```python
from build123d import *

# Parameters (mm, degrees)
SKETCH1_R           = 23.5
BOSS_EXTRUDE1_DEPTH = 65
SKETCH2_R           = 7.5
BOSS_EXTRUDE2_DEPTH = 2
SKETCH3_R           = 2.5
BOSS_EXTRUDE3_DEPTH = 20
CUT_EXTRUDE2_START  = -7.5
CUT_EXTRUDE2_DEPTH  = 7.5


with BuildPart() as part:
    # Sketch1 → Boss-Extrude1 (new body)
    with BuildSketch(Plane(origin=(0, 0, 0), x_dir=(1, 0, 0), z_dir=(0, 1, 0))):
        with Locations(Location((0, 0, 0), (0, 0, 270))):
            Circle(SKETCH1_R)
    extrude(amount=BOSS_EXTRUDE1_DEPTH)

    # Sketch2 → Boss-Extrude2 (add)
    with BuildSketch(Plane(origin=(0, 65, 0), x_dir=(1, 0, 0), z_dir=(0, 1, 0))):
        with Locations(Location((0, 0, 0), (0, 0, 270))):
            Circle(SKETCH2_R)
    extrude(amount=BOSS_EXTRUDE2_DEPTH)

    # Sketch3 → Boss-Extrude3 (add)
    with BuildSketch(Plane(origin=(0, 67, 0), x_dir=(1, 0, 0), z_dir=(0, 1, 0))):
        with Locations(Location((0, 0, 0), (0, 0, 270))):
            Circle(SKETCH3_R)
    extrude(amount=BOSS_EXTRUDE3_DEPTH)

    # Sketch4 → Cut-Extrude2 (cut)
    with BuildSketch(Plane(origin=(0, 87, 0), x_dir=(1, 0, 0), z_dir=(0, 1, 0)).offset(CUT_EXTRUDE2_START)):
        with BuildLine():
            Line((0.591953549, 2.428907367), (0.591953549, -2.428907367))
            ThreePointArc((0.591953549, -2.428907367), (2.5, 0), (0.591953549, 2.428907367))
        make_face()
    extrude(amount=CUT_EXTRUDE2_DEPTH, mode=Mode.SUBTRACT)


solid = part.part
```
Check sheet for the modelled part. Datum: model origin and axes. Units: mm. A direction names the side the tool comes from. Round coordinates to 2 decimals unless told otherwise and drop trailing zeros. Write each loop counter-clockwise with the first axis right and the second up, starting at its lowest first coordinate (ties: lowest second). Pieces come first, ordered by that corner, then holes. Notation, with made-up numbers: M -6,60.25 L 25,60.25 A25 cw 25,81.25 Z; hole C -25,-22 d8. An arc over 180 degrees is marked long. Write item = value, one per line. Start each with the question number.
1. Section check B-B, the plane y = 80.5. Record the cut outline in (x, z).
2. Section check C-C, the plane y = 6. Record the cut outline in (x, z), then the cut area to 3 significant figures.
3. Gauge pin test, flat ends, axial feed: pin 1 (2 mm diameter, centred on x = -3.5, y = 14.5, fed in from -Z); pin 2 (2 mm diameter, centred on x = -2, y = 78, fed in from -Z); pin 3 (23.5 mm diameter, centred on x = 1, z = 2.5, fed in from +Y); pin 4 (8 mm diameter, centred on x = 12, z = 3.5, fed in from +Y). Record the tip position at first contact, or that the pin passes through.
4. Scan lines: line 1 (Y direction, x = -5.5, z = 7.5); line 2 (Z direction, x = 0.5, y = 13). Record each from-to range of solid material in increasing order. Write a range as [from, to].
5. Tool access check on faces 1 (the cylindrical face through (15.88, 32.04, -17.32)), 2 (the cylindrical face through (-2.44, 74.64, -0.54)), 3 (the flat face through (0.592, 83, 0)). Record the directions out of +Z, -Z, +X, -X, +Y, -Y that give a thin tool (end or side, any length) a straight path to the whole face; none if there is none.
6. Section check A-A, the plane z = 0. Record the cut outline in (x, y).
7. Section check D-D, the plane x = 20. Record the cut outline in (y, z), then the cut area to 3 significant figures.
Results found:
q1.outline = M 0.59,-2.43 L 0.59,2.43 A2.5 ccw long Z
q2.outline = C 0,0 d47
q2.area = 1,730 mm^2
q3.pin_1 = -23.37
q3.pin_2 = -2.29
q3.pin_3 = 87
q3.pin_4 = 65
q4.line_1 = [0, 65]
q4.line_2 = [-23.49, 23.49]
q5.face_1 = +Y, -Y
q5.face_2 = +Y
q5.face_3 = +Z, -Z, +X, +Y
q6.outline = M -23.5,0 L 23.5,0 L 23.5,65 L 7.5,65 L 7.5,67 L 2.5,67 L 2.5,79.5 L 0.59,79.5 L 0.59,87 L -2.5,87 L -2.5,67 L -7.5,67 L -7.5,65 L -23.5,65 Z
q7.outline = M 0,-12.34 L 65,-12.34 L 65,12.34 L 0,12.34 Z
q7.area = 1,600 mm^2
